The listing builds one solid part. Answer for the finished solid, in the listing's coordinates (mm). A direction names the side the tool comes from. Coordinates: 2 decimals unless noted, no trailing zeros. Order: outer loops, then holes, each group sorted by start corner. A loop starts at its lowest first (then second) coordinate and runs counter-clockwise, first axis right, second up. Notation, with made-up numbers: (-17, 7.5) - (6, 7.5) arc R25 ccw to (6, 39.5) - close; hole circle Ø9 at (65.25, -38.75). An arc over 180 degrees is marked (long way). Use one line per item in the form item = value. Start each with the question number.
Item 1: Section A-A, the plane x = 7.75 is taken. Write down the section's boundary in (y, z).
Item 2: Consider line 1 along Y through (x, z) = (4, 15); line 2 along Z through (x, y) = (2.75, 7.5); line 3 along Y through (x, z) = (7, -15). Determine where each line is inside the solid, lowest interval first. Write a range as [from, to].
Item 3: A tool of negligible diameter and unlimited length cuts with its end or side. For faces 4 (the flat face through (6.5, -6.5, 5.7)), 5 (the flat face through (5, -8, 4.862)), 6 (the flat face through (1, 6, -9)), from which of +Z, -Z, +X, -X, +Y, -Y can it reach the whole face along a straight path? Write none if from no direction.
Item 4: Section C-C, the plane y = -4 is taken. Write down the section's boundary in (x, z).
Item 5: Section B-B, the plane y = 8 is taken. Write down the section's boundary in (x, z).
Item 6: Section D-D, the plane z = 14 is taken. Write down the section's boundary in (x, y), and give its area (3 significant figures).
Item 7: The mould has two halves that part along Z. Classify faces 1 (the flat face through (3, 7, -8)), 2 (the cylindrical face through (4.93, 21.48, -0.91)), 3 (the flat face through (0, -1, -12)): released by +Z, released by -Z, zero draft, split by the parting line, or undercut.
Item 8: Each of these flat-tipped pins is pushed along its axis until it touches: pin 1 Ø1 at (x, y) = (7.5, -16) entering from +Z; pin 2 Ø1.9 at (x, z) = (8.5, 6) entering from +Y; pin 3 Ø3 at (x, y) = (5, -14.5) entering from -Z. Where does it stop, or does it pass through?
from build123d import *

# Parameters (mm, degrees)
SKETCH1_R           = 21.5
BOSS_EXTRUDE1_DEPTH = 10
CUT_EXTRUDE2_DEPTH  = 10
SKETCH15_W          = 18
SKETCH15_H          = 24.118038922
CUT_EXTRUDE3_DEPTH  = 3
SKETCH17_W          = 4
SKETCH17_H          = 1.75
BOSS_EXTRUDE3_DEPTH = 1
SKETCH18_W          = 6.5
SKETCH18_H          = 1.737607108
BOSS_EXTRUDE4_DEPTH = 1
SKETCH39_W          = 2.4
SKETCH39_H          = 4.126590585
CUT_EXTRUDE7_DEPTH  = 3
SKETCH41_R          = 1.75
SKETCH41_R_2        = 2.1
CUT_EXTRUDE8_DEPTH  = 11


with BuildPart() as part:
    # Sketch1 → Boss-Extrude1 (new body)
    with BuildSketch(Plane(origin=(0, 0, 0), x_dir=(0, 0, -1), z_dir=(1, 0, 0))):
        Circle(SKETCH1_R)
    extrude(amount=BOSS_EXTRUDE1_DEPTH)

    # Sketch13 → Cut-Extrude2 (cut)
    with BuildSketch(Plane(origin=(0, 0, 0), x_dir=(0, 0, -1), z_dir=(1, 0, 0))):
        with BuildLine():
            Line((-2.670420152, -16.85816067), (-2.770420152, -16.530371213))
            Line((-2.770420152, -16.530371213), (-4.862392892, -10))
            Line((-4.862392892, -10), (-4.862392892, -6.943148259))
            Line((-4.862392892, -6.943148259), (-6.6, -6.943148259))
            Line((-6.6, -6.943148259), (-6.6, 19.556851741))
            Line((-6.6, 19.556851741), (6.6, 19.556851741))
            Line((6.6, 19.556851741), (6.6, -6.943148259))
            Line((6.6, -6.943148259), (4.862392892, -6.943148259))
            Line((4.862392892, -6.943148259), (4.862392892, -10))
            Line((4.862392892, -10), (2.770420152, -16.530371213))
            Line((2.770420152, -16.530371213), (2.670420152, -16.85816067))
            Line((2.670420152, -16.85816067), (2.670420152, -21.837327131))
            ThreePointArc((2.670420152, -21.837327131), (1.836835043, -21.92318492), (1.000584871, -21.977234355))
            Line((1.000584871, -21.977234355), (0, -25.25))
            Line((0, -25.25), (-1.000584871, -21.977234355))
            ThreePointArc((-1.000584871, -21.977234355), (-1.836835043, -21.92318492), (-2.670420152, -21.837327131))
            Line((-2.670420152, -21.837327131), (-2.670420152, -16.85816067))
        make_face()
    extrude(amount=CUT_EXTRUDE2_DEPTH, mode=Mode.SUBTRACT)

    # Sketch15 → Cut-Extrude3 (cut)
    with BuildSketch(Plane.ZY):
        with Locations((0, 5.115871202)):
            Rectangle(SKETCH15_W, SKETCH15_H)
    extrude(amount=-CUT_EXTRUDE3_DEPTH, mode=Mode.SUBTRACT)

    # Sketch17 → Boss-Extrude3 (add)
    with BuildSketch(Plane(origin=(0, -6.943148259, 0), x_dir=(1, 0, 0), z_dir=(0, 1, 0))):
        with Locations((2, 5.737392892)):
            Rectangle(SKETCH17_W, SKETCH17_H)
    extrude(amount=BOSS_EXTRUDE3_DEPTH)

    # Sketch18 → Boss-Extrude4 (add)
    with BuildSketch(Plane(origin=(0, -6.943148259, 0), x_dir=(1, 0, 0), z_dir=(0, 1, 0))):
        with Locations((3.25, -5.731196446)):
            Rectangle(SKETCH18_W, SKETCH18_H)
    extrude(amount=BOSS_EXTRUDE4_DEPTH)

    # Sketch39 → Cut-Extrude7 (cut)
    with BuildSketch(Plane(origin=(0, 0, 0), x_dir=(0, 0, -1), z_dir=(1, 0, 0))):
        with Locations((7.8, 19.238185956)):
            Rectangle(SKETCH39_W, SKETCH39_H)
        with Locations((-7.8, 19.238185956)):
            Rectangle(SKETCH39_W, SKETCH39_H)
    extrude(amount=CUT_EXTRUDE7_DEPTH, mode=Mode.SUBTRACT)

    # Sketch41 → Cut-Extrude8 (cut, through all)
    with BuildSketch(Plane.ZY):
        with Locations((-15, 8)):
            Circle(SKETCH41_R)
        with Locations((15, 8)):
            Circle(SKETCH41_R)
        with Locations((15, -8)):
            Circle(SKETCH41_R)
        with Locations((-15, -8)):
            Circle(SKETCH41_R)
        with Locations((-15, 0)):
            Circle(SKETCH41_R_2)
    extrude(amount=-CUT_EXTRUDE8_DEPTH, mode=Mode.SUBTRACT)


solid = part.part
Response:
q1.outline = (-21.33, -2.67) arc R21.5 ccw (long way) to (-21.33, 2.67) - (-16.86, 2.67) - (-16.53, 2.77) - (-10, 4.86) - (-6.94, 4.86) - (-6.94, 6.6) - (19.56, 6.6) - (19.56, -6.6) - (-6.94, -6.6) - (-6.94, -4.86) - (-10, -4.86) - (-16.53, -2.77) - (-16.86, -2.67) - close; hole circle Ø3.5 at (-8, -15); hole circle Ø3.5 at (-8, 15); hole circle Ø4.2 at (0, -15); hole circle Ø3.5 at (8, -15); hole circle Ø3.5 at (8, 15)
q2.line_1 = [-15.4, -9.75], [-6.25, 6.25], [9.75, 15.4]
q2.line_2 = [-20.15, -16.68], [-13.32, -9], [9, 13.32], [16.68, 20.15]
q2.line_3 = [-15.4, -9.75], [-6.25, -2.1], [2.1, 6.25], [9.75, 15.4]
q3.face_4 = +X
q3.face_5 = +X, -X
q3.face_6 = -X, +Y
q4.outline = (0, -21.12) - (10, -21.12) - (10, -6.6) - (3, -6.6) - (3, -9) - (0, -9) - close; (0, 9) - (3, 9) - (3, 6.6) - (10, 6.6) - (10, 21.12) - (0, 21.12) - close
q5.outline = (0, -19.96) - (10, -19.96) - (10, -16.75) - (0, -16.75) - close; (0, -13.25) - (10, -13.25) - (10, -6.6) - (3, -6.6) - (3, -9) - (0, -9) - close; (0, 9) - (3, 9) - (3, 6.6) - (10, 6.6) - (10, 13.25) - (0, 13.25) - close; (0, 16.75) - (10, 16.75) - (10, 19.96) - (0, 19.96) - close
q6.outline = (0, -16.32) - (10, -16.32) - (10, -9.44) - (0, -9.44) - close; (0, -6.56) - (10, -6.56) - (10, 6.56) - (0, 6.56) - close; (0, 9.44) - (10, 9.44) - (10, 16.32) - (0, 16.32) - close
q6.area = 269 mm2
q7.face_1 = undercut
q7.face_2 = split by the parting line
q7.face_3 = zero draft
q8.pin_1 = 14.9
q8.pin_2 = 20.9
q8.pin_3 = -17.12
